The listing builds one solid part. Answer for the finished solid, in the listing's coordinates (mm). Face numbers are marked on the shaded views. Coordinates: 2 decimals unless noted, no trailing zeros. Loops run counter-clockwise (first coordinate to the right, second up) from the corner with the lowest first, then second, coordinate; pieces in that order, holes last. Notation, with made-up numbers: (-37.75, 57) - (17.25, 57) arc R19 cw to (17.25, 82) - close; hole circle Ø11 at (-19.5, 33.25). An arc over 180 degrees is marked (long way). Return JSON: item names as keys, results as strings. Group by question number.
1. The mould has two halves that part along Z. Classify the marked faces 1 and 2: pulls with the +Z half, pulls with the -Z half, needs draft (parallel to the pull), parting line crosses it, or undercut.
2. Section D-D (y = 0.5) is taken. Write down the section's boundary in (x, z), and give its area (3 significant figures).
3. Section C-C (z = 30.5) is taken. Write down the section's boundary in (x, y) (3 decimals).
4. Section A-A (z = 19.5) is taken. Write down the section's boundary in (x, y) (3 decimals), and give its area (3 significant figures).
5. Find the intervals of material crossed by line 1 along Y through (x, z) = (2.5, 36.5) (3 decimals); line 2 along Z through (x, y) = (-20.5, -2.5); line 3 along Z through (x, y) = (-11, 1), in increasing order.
6. Section B-B (x = 18.5) is taken. Write down the section's boundary in (y, z) (3 decimals).
```python
from build123d import *

# Parameters (mm, degrees)
F0_W          = 152.4
F0_H          = 31.75
F1_DEPTH      = 57.15
F3_DEPTH      = 5.55625
F3_DEPTH_BACK = 5.55625
F4_DEPTH      = 6.35
F5_R          = 2.54
F6_T1_DEPTH   = 60.96
F6_S5_W       = 2.54
F6_S5_H       = 2.54
F6_T6_DEPTH   = 2.54
F6_S11_W      = 2.54
F6_S11_H      = 2.54
F6_T12_DEPTH  = 2.54


# Not quite as in the source:
# - a fillet or chamfer that OpenCascade refuses, or shapes differently, is made with other operations: its cross-section is extruded or revolved along the edge and cut away or added


with BuildPart() as f1:
    # F0 (on Top) → F1 (new body)
    with BuildSketch(Plane.XY):
        Rectangle(F0_W, F0_H)
    extrude(amount=F1_DEPTH)

    # F2 (on Front) → F3 (cut, two sides)
    with BuildSketch(Plane.XZ) as f3_sk:
        with BuildLine():
            Line((76.2, 57.2062885404), (0, 57.2062885404))
            Line((0, 57.2062885404), (-76.2, 57.2062885404))
            ThreePointArc((-76.2, 57.2062885404), (-5.9418927192, 12.810203488), (76.2, 25.4562885404))
            Line((76.2, 25.4562885404), (76.2, 57.2062885404))
        make_face()
    extrude(amount=F3_DEPTH, mode=Mode.SUBTRACT)
    extrude(f3_sk.sketch, amount=-F3_DEPTH_BACK, mode=Mode.SUBTRACT)

    # F4 (add): a face of the model
    f4_faces = [f1.faces().sort_by_distance(p)[0] for p in [
        (-76.2, 0, 28.575),
    ]]
    extrude(f4_faces, amount=F4_DEPTH)

    # F5
    f5_edges = [f1.edges().sort_by_distance(p)[0] for p in [
        (76.2, -10.715625, 57.15),
        (-3.175, -15.875, 57.15),
        (76.2, -15.875, 28.575),
        (76.2, 10.715625, 57.15),
        (76.2, 15.875, 28.575),
        (-3.175, 15.875, 57.15),
        (-82.55, 0, 57.15),
        (0.021369, -5.55625, 57.15),
        (-76.157263, 0, 57.15),
        (0.021369, 5.55625, 57.15),
        (76.2, 5.55625, 41.303144),
        (76.2, -5.55625, 41.303144),
        (76.2, 0, 25.456289),
    ]]
    fillet(f5_edges, radius=F5_R)

    # F6: fillet of radius 2.54 on 2 edges, made by hand

    # F6_s2 → F6_t1 (cut)
    with BuildSketch(Plane.XY.offset(-6.35)):
        with BuildLine():
            ThreePointArc((-80.01, 15.875), (-81.8060512242, 15.1310512242), (-82.55, 13.335))
            Line((-82.55, 13.335), (-82.55, 15.875))
            Line((-82.55, 15.875), (-80.01, 15.875))
        make_face()
        with BuildLine():
            ThreePointArc((-82.55, -13.335), (-81.8060512242, -15.1310512242), (-80.01, -15.875))
            Line((-80.01, -15.875), (-82.55, -15.875))
            Line((-82.55, -15.875), (-82.55, -13.335))
        make_face()
    extrude(amount=F6_T1_DEPTH, mode=Mode.SUBTRACT)


with BuildPart() as f6_tool4:
    # F6_s5 → F6_t6 (new body)
    with BuildSketch(Plane.YZ.offset(-80.01)):
        with Locations((-14.605, 55.88)):
            Rectangle(F6_S5_W, F6_S5_H)
    extrude(amount=-F6_T6_DEPTH)

    # F6_s7 → F6_t8 (revolve, cut)
    with BuildSketch(Plane(origin=(-80.01, -13.335, 54.61), x_dir=(0, 0.7071067812, -0.7071067812), z_dir=(0, 0.7071067812, 0.7071067812))):
        with BuildLine():
            ThreePointArc((0, -2.54), (2.54, 0), (0, 2.54))
            Line((0, 2.54), (0, -2.54))
        make_face()
    revolve(axis=Axis((-80.01, -13.335, 54.61), (-1, 0, 0)), mode=Mode.SUBTRACT)


with BuildPart() as f1_1:
    add(f1.part)

    # F6_t3: cut F6_tool4
    add(f6_tool4.part, mode=Mode.SUBTRACT)


with BuildPart() as f6_tool10:
    # F6_s11 → F6_t12 (new body)
    with BuildSketch(Plane.XZ.offset(-13.335)):
        with Locations((-81.28, 55.88)):
            Rectangle(F6_S11_W, F6_S11_H)
    extrude(amount=-F6_T12_DEPTH)

    # F6_s13 → F6_t14 (revolve, cut)
    with BuildSketch(Plane(origin=(-80.01, 13.335, 54.61), x_dir=(0.7071067812, 0, -0.7071067812), z_dir=(0.7071067812, 0, 0.7071067812))):
        with BuildLine():
            ThreePointArc((0, -2.54), (2.54, 0), (0, 2.54))
            Line((0, 2.54), (0, -2.54))
        make_face()
    revolve(axis=Axis((-80.01, 13.335, 54.61), (0, 1, 0)), mode=Mode.SUBTRACT)


with BuildPart() as f1_2:
    add(f1_1.part)

    # F6_t9: cut F6_tool10
    add(f6_tool10.part, mode=Mode.SUBTRACT)


solid = f1_2.part
```
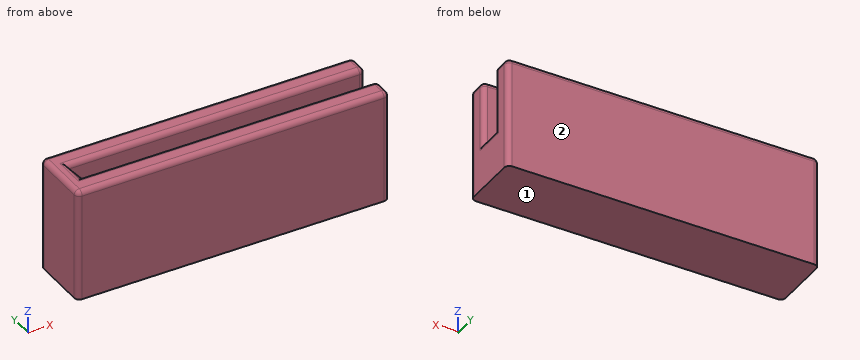
The answers:
{
 "1": {"face 1": "pulls with the -Z half", "face 2": "needs draft"},
 "2": {"outline": "(-82.55, 0) - (76.2, 0) - (76.2, 21.21) arc R2.54 ccw to (72.5, 23.47) arc R118.54 cw to (-75.4, 56.17) arc R2.54 ccw to (-77.41, 57.15) - (-80.01, 57.15) arc R2.54 ccw to (-82.55, 54.61) - close", "area": "3,550 mm2"},
 "3": {"outline": "(-82.55, -13.335) arc R2.54 ccw to (-80.01, -15.875) - (73.66, -15.875) arc R2.54 ccw to (76.2, -13.335) - (76.2, -8.096) arc R2.54 ccw to (73.66, -5.556) - (-47.927, -5.556) - (-47.927, 5.556) - (73.66, 5.556) arc R2.54 ccw to (76.2, 8.096) - (76.2, 13.335) arc R2.54 ccw to (73.66, 15.875) - (-80.01, 15.875) arc R2.54 ccw to (-82.55, 13.335) - close"},
 "4": {"outline": "(-82.55, -13.335) arc R2.54 ccw to (-80.01, -15.875) - (73.66, -15.875) arc R2.54 ccw to (76.2, -13.335) - (76.2, 13.335) arc R2.54 ccw to (73.66, 15.875) - (-80.01, 15.875) arc R2.54 ccw to (-82.55, 13.335) - close; hole (-27.509, -5.556) - (63.98, -5.556) - (63.98, 5.556) - (-27.509, 5.556) - close", "area": "4,020 mm2"},
 "5": {"line 1": "y = -15.875 to -5.556, 5.556 to 15.875", "line 2": "z = 0 to 16.83", "line 3": "z = 0 to 13.98"},
 "6": {"outline": "(-15.875, 0) - (15.875, 0) - (15.875, 54.61) arc R2.54 ccw to (13.335, 57.15) - (8.096, 57.15) arc R2.54 ccw to (5.556, 54.61) - (5.556, 10.319) - (-5.556, 10.319) - (-5.556, 54.61) arc R2.54 ccw to (-8.096, 57.15) - (-13.335, 57.15) arc R2.54 ccw to (-15.875, 54.61) - close"}
}
